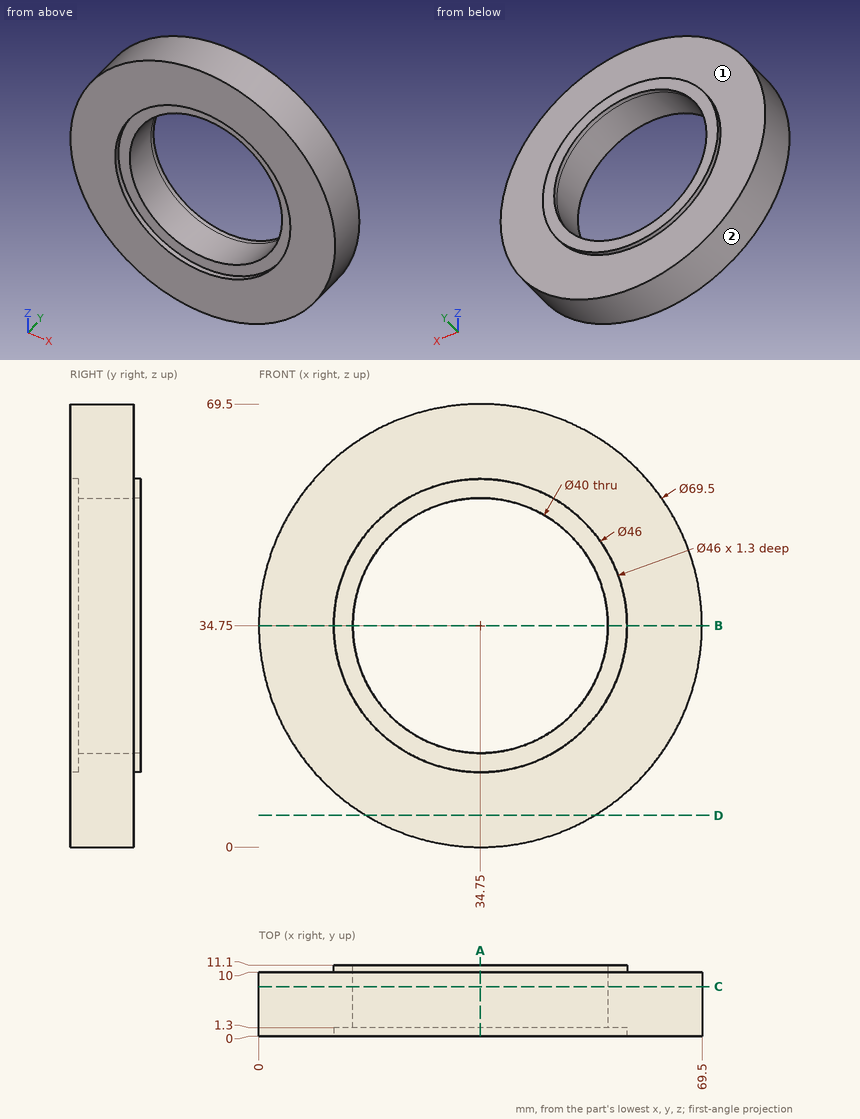
Source: three-view drawing plus pictorial views. Frame: mm from the lowest corner of the part. Round coordinates to 2 decimals unless told otherwise and drop trailing zeros. Order: outer loops, then holes, each group sorted by start corner. A loop starts at its lowest first (then second) coordinate and runs counter-clockwise, first axis right, second up. Notation, with made-up numbers: (39, -33) -> (70, -33) arc R23 cw to (70, -24) -> close; hole circle Ø9 at (34.5, 74.25). An arc over 180 degrees is marked (long way). Use CSV: the item, a comma, the result in double quotes. Start each with the question number.
1) Section A-A (x = 34.75). Return the cut outline in (y, z).
2) First-contact query: pin 1 Ø1.5 at (y, z) = (7.5, 21.5) entering from +X; pin 2 Ø5 at (x, y) = (53, 5) entering from -Z; pin 3 Ø8 at (x, z) = (22.5, 33) entering from -Y; pin 4 Ø1.5 at (y, z) = (6.5, 60.5) entering from +X. Flat tips, straight axial feed; report the tip coordinate or a pass-through.
3) Draft query along Z for the marked faces 1 and 2. Return one class per face: +Z half, -Z half, draft (parallel to the pull), parting line (faces both ways), or undercut.
4) Section C-C (y = 7.75). Return the cut outline in (x, z).
5) Section B-B (z = 34.75). Return the cut outline in (x, y).
6) Section D-D (z = 5). Return the cut outline in (x, y).
7) Material intervals for line 1 along Z through (x, y) = (34.75, 5.5); line 2 along X through (y, z) = (4, 34); line 3 along Z through (x, y) = (34.75, 0.5), sorted ascending. Write a range as from..to.
Returned:
1,outline,"(0, 0) -> (10, 0) -> (10, 11.75) -> (11.1, 11.75) -> (11.1, 14.75) -> (1.3, 14.75) -> (1.3, 11.75) -> (0, 11.75) -> close; (0, 57.75) -> (1.3, 57.75) -> (1.3, 54.75) -> (11.1, 54.75) -> (11.1, 57.75) -> (10, 57.75) -> (10, 69.5) -> (0, 69.5) -> close"
2,pin 1,"stops at x = 67.17"
2,pin 2,"stops at z = 3.77"
2,pin 3,"passes through"
2,pin 4,"stops at x = 58.89"
3,face 1,"draft"
3,face 2,"parting line"
4,outline,"circle Ø69.5 at (34.75, 34.75); hole circle Ø40 at (34.75, 34.75)"
5,outline,"(0, 0) -> (11.75, 0) -> (11.75, 1.3) -> (14.75, 1.3) -> (14.75, 11.1) -> (11.75, 11.1) -> (11.75, 10) -> (0, 10) -> close; (54.75, 1.3) -> (57.75, 1.3) -> (57.75, 0) -> (69.5, 0) -> (69.5, 10) -> (57.75, 10) -> (57.75, 11.1) -> (54.75, 11.1) -> close"
6,outline,"(16.79, 0) -> (52.71, 0) -> (52.71, 10) -> (16.79, 10) -> close"
7,line 1,"z = 0..14.75, 54.75..69.5"
7,line 2,"x = 0.01..14.76, 54.74..69.49"
7,line 3,"z = 0..11.75, 57.75..69.5"
